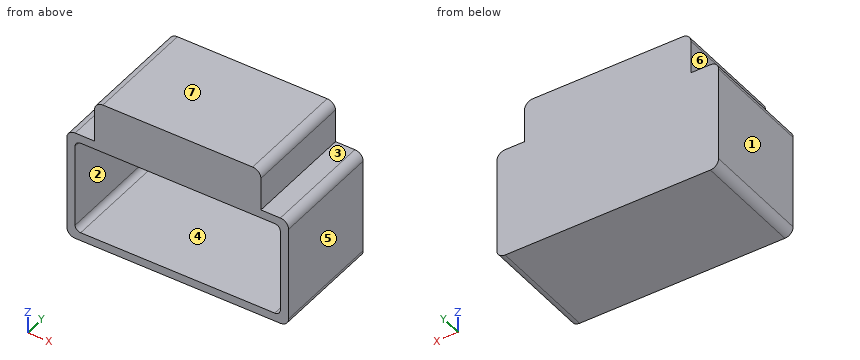
```python
from build123d import *

# Parameters (mm, degrees)
F1_DEPTH = 50.8
F2_T     = 3.81
F3_R     = 2.54
F4_DEPTH = 50.8


# Not quite as in the source:
# - a shell that OpenCascade refuses in one call is made with other operations: the cavity is built on its own and cut out


with BuildPart() as f1:
    # F0 (on Front) → F1 (new body)
    with BuildSketch(Plane.XZ):
        with BuildLine():
            ThreePointArc((50.8, 21.59), (49.6840768363, 24.2840768363), (46.99, 25.4))
            Line((46.99, 25.4), (38.1, 25.4))
            Line((38.1, 25.4), (-38.1, 25.4))
            Line((-38.1, 25.4), (-46.99, 25.4))
            ThreePointArc((-46.99, 25.4), (-49.6840768363, 24.2840768363), (-50.8, 21.59))
            Line((-50.8, 21.59), (-50.8, -21.59))
            ThreePointArc((-50.8, -21.59), (-49.6840768363, -24.2840768363), (-46.99, -25.4))
            Line((-46.99, -25.4), (46.99, -25.4))
            ThreePointArc((46.99, -25.4), (49.6840768363, -24.2840768363), (50.8, -21.59))
            Line((50.8, -21.59), (50.8, 21.59))
        make_face()
    extrude(amount=F1_DEPTH)

    # F2: shell of thickness 3.81, made by hand


with BuildPart() as f2_core1:
    # F2_t2: copy of F1
    add(f1.part)

    # the walls: a layer under each face that stays
    f2_faces = [f2_core1.faces().sort_by_distance(p)[0] for p in [
        (0, -25.4, -25.4),
        (-50.8, -25.4, 0),
        (0, 0, 0),
        (0, -25.4, 25.4),
        (50.8, -25.4, 0),
    ]]
    thicken(f2_faces, amount=-F2_T, mode=Mode.SUBTRACT)


with BuildPart() as f1_1:
    add(f1.part)

    # what is left inside the walls is the cavity
    f2_cavity = [f2_core1.part.solids().sort_by_distance(p)[0] for p in [
        (0, -35.136667, -21.5519),
    ]]
    add(f2_cavity, mode=Mode.SUBTRACT)

    # F3
    f3_edges = [f1_1.edges().sort_by_distance(p)[0] for p in [
        (-46.99, -27.305, 21.59),
        (-46.99, -27.305, -21.59),
        (46.99, -27.305, -21.59),
        (46.99, -27.305, 21.59),
    ]]
    fillet(f3_edges, radius=F3_R)

    # F0 (on Front) → F4 (join)
    with BuildSketch(Plane.XZ):
        with BuildLine():
            Line((-38.1, 25.4), (38.1, 25.4))
            Line((38.1, 25.4), (38.1, 40.64))
            ThreePointArc((38.1, 40.64), (36.9840768363, 43.3340768363), (34.29, 44.45))
            Line((34.29, 44.45), (0, 44.45))
            Line((0, 44.45), (-34.29, 44.45))
            ThreePointArc((-34.29, 44.45), (-36.9840768363, 43.3340768363), (-38.1, 40.64))
            Line((-38.1, 40.64), (-38.1, 25.4))
        make_face()
    extrude(amount=F4_DEPTH)


solid = f1_1.part
```
Here's how the part is built. I have some questions about the finished solid (model axes, mm). Face numbers are marked on the shaded views. A direction names the side the tool comes from. Give positions to 0.01 mm unless a question says otherwise; leave off trailing zeros. Loops run counter-clockwise (first coordinate to the right, second up) from the corner with the lowest first, then second, coordinate; pieces in that order, holes last. Notation, with made-up numbers: M -18,82 L 33,82 A13 ccw 33,95 Z; hole C -34.75,17.5 d6. An arc over 180 degrees is marked long. Put each result on its own line as item: value. Start each with the question number.
(1) If we mould it in two halves opening along X, with no side actions, what happens to the marked faces 4, 5, 6 and 7? For each: +X half, -X half, draft (parallel to the pull), parting line (faces both ways), or undercut.
(2) I want a section at C-C on x = 19.5. Please give me the cut outline in (y, z), then the cut area to 3 significant figures.
(3) I want a section at A-A on y = -6. Please give me the cut outline in (x, z), then the cut area to 3 significant figures.
(4) I need wall thicknesses on line 1 along Z through (x, y) = (-6.5, -4); line 2 along X through (y, z) = (-9.5, 18); line 3 along Z through (x, y) = (-39.5, -40). Which ranges of each line are inside material? Lowest first, please. Write a range as [from, to].
(5) For the marked faces 1, 2 and 3, which set-ups out of +Z, -Z, +X, -X, +Y, -Y let a thin tool reach every point of the face, with its end or its side?
(6) I want a section at B-B on z = 2.5. Please give me the cut outline in (x, y), then the cut area to 3 significant figures.
(7) Will these pins go through, and if not, where does the flat tip stop? pin 1 Ø2.5 at (x, y) = (-42, -24.5) entering from +Z; pin 2 Ø7.5 at (y, z) = (-34, 29.5) entering from -X; pin 3 Ø2 at (y, z) = (-13.5, 30) entering from +X.
(8) I want a section at D-D on z = 29. Please give me the cut outline in (x, y).
Answer block:
1. face 4: undercut
1. face 5: +X half
1. face 6: -X half
1. face 7: draft
2. outline: M -50.8,-25.4 L 0,-25.4 L 0,44.45 L -50.8,44.45 L -50.8,21.59 L -3.81,21.59 L -3.81,-21.59 L -50.8,-21.59 Z
2. area: 1,520 mm^2
3. outline: M -50.8,-21.59 A3.81 ccw -46.99,-25.4 L 46.99,-25.4 A3.81 ccw 50.8,-21.59 L 50.8,21.59 A3.81 ccw 46.99,25.4 L 38.1,25.4 L 38.1,40.64 A3.81 ccw 34.29,44.45 L -34.29,44.45 A3.81 ccw -38.1,40.64 L -38.1,25.4 L -46.99,25.4 A3.81 ccw -50.8,21.59 Z; hole M -46.99,-19.05 A2.54 ccw -44.45,-21.59 L 44.45,-21.59 A2.54 ccw 46.99,-19.05 L 46.99,19.05 A2.54 ccw 44.45,21.59 L -44.45,21.59 A2.54 ccw -46.99,19.05 Z
3. area: 2,540 mm^2
4. line 1: [-25.4, -21.59], [21.59, 44.45]
4. line 2: [-50.8, -46.99], [46.99, 50.8]
4. line 3: [-25.4, -21.59], [21.59, 25.4]
5. face 1: +Z, -Z, -X, +Y, -Y
5. face 2: -Y
5. face 3: +Z, +X, +Y, -Y
6. outline: M -50.8,-50.8 L -46.99,-50.8 L -46.99,-3.81 L 46.99,-3.81 L 46.99,-50.8 L 50.8,-50.8 L 50.8,0 L -50.8,0 Z
6. area: 745 mm^2
7. pin 1: z = 25.4
7. pin 2: x = -38.1
7. pin 3: x = 38.1
8. outline: M -38.1,-50.8 L 38.1,-50.8 L 38.1,0 L -38.1,0 Z
